```python
from build123d import *

# Parameters (mm, degrees)
BOSS_EXTRUDE1_DEPTH = 6.35
SKETCH2_R           = 2.4892
SKETCH2_R_2         = 4.7625
CUT_EXTRUDE1_DEPTH  = 7.35
FILLET1_R           = 6.35


with BuildPart() as part:
    # Sketch1 → Boss-Extrude1 (new body)
    with BuildSketch(Plane(origin=(0, 0, 0), x_dir=(1, 0, 0), z_dir=(0, 1, 0))):
        Polygon((0, 95.812682967), (85.38707615, 217.758065572), (127, 188.620382605), (127, 0), (0, 0), align=None)
    extrude(amount=BOSS_EXTRUDE1_DEPTH)

    # Sketch2 → Cut-Extrude1 (cut, through all)
    with BuildSketch(Plane(origin=(0, 6.35, 0), x_dir=(1, 0, 0), z_dir=(0, 1, 0))):
        with Locations((12.7, 12.7)):
            Circle(SKETCH2_R)
        with Locations((12.7, 38.1)):
            Circle(SKETCH2_R)
        with Locations((25.4, 38.1)):
            Circle(SKETCH2_R)
        with Locations((38.1, 38.1)):
            Circle(SKETCH2_R)
        with Locations((50.8, 38.1)):
            Circle(SKETCH2_R)
        with Locations((63.5, 38.1)):
            Circle(SKETCH2_R)
        with Locations((25.4, 12.7)):
            Circle(SKETCH2_R)
        with Locations((38.1, 12.7)):
            Circle(SKETCH2_R)
        with Locations((50.8, 12.7)):
            Circle(SKETCH2_R)
        with Locations((63.5, 12.7)):
            Circle(SKETCH2_R)
        with Locations((76.2, 12.7)):
            Circle(SKETCH2_R)
        with Locations((76.2, 38.1)):
            Circle(SKETCH2_R)
        with Locations((88.9, 12.7)):
            Circle(SKETCH2_R)
        with Locations((88.9, 38.1)):
            Circle(SKETCH2_R)
        with Locations((101.6, 12.7)):
            Circle(SKETCH2_R)
        with Locations((101.6, 38.1)):
            Circle(SKETCH2_R)
        with Locations((90.531859121, 202.963802812)):
            Circle(SKETCH2_R)
        with Locations((111.338321046, 188.394961329)):
            Circle(SKETCH2_R)
        with Locations((83.247438379, 192.56057185)):
            Circle(SKETCH2_R)
        with Locations((104.053900304, 177.991730366)):
            Circle(SKETCH2_R)
        with Locations((75.963017637, 182.157340887)):
            Circle(SKETCH2_R)
        with Locations((96.769479562, 167.588499404)):
            Circle(SKETCH2_R)
        with Locations((68.678596896, 171.754109925)):
            Circle(SKETCH2_R)
        with Locations((89.485058821, 157.185268441)):
            Circle(SKETCH2_R)
        with Locations((61.394176154, 161.350878962)):
            Circle(SKETCH2_R)
        with Locations((82.200638079, 146.782037479)):
            Circle(SKETCH2_R)
        with Locations((54.109755412, 150.947648)):
            Circle(SKETCH2_R)
        with Locations((74.916217337, 136.378806516)):
            Circle(SKETCH2_R)
        with Locations((46.825334671, 140.544417037)):
            Circle(SKETCH2_R)
        with Locations((67.631796596, 125.975575554)):
            Circle(SKETCH2_R)
        with Locations((39.540913929, 130.141186075)):
            Circle(SKETCH2_R)
        with Locations((60.347375854, 115.572344592)):
            Circle(SKETCH2_R)
        with Locations((17.687651704, 98.931493187)):
            Circle(SKETCH2_R_2)
        with Locations((28.090882667, 91.647072446)):
            Circle(SKETCH2_R_2)
        with Locations((38.494113629, 84.362651704)):
            Circle(SKETCH2_R_2)
        with Locations((114.3, 12.7)):
            Circle(SKETCH2_R)
        with Locations((114.3, 38.1)):
            Circle(SKETCH2_R)
    extrude(amount=-CUT_EXTRUDE1_DEPTH, mode=Mode.SUBTRACT)

    # Fillet1
    fillet1_edges = [part.edges().sort_by_distance(p)[0] for p in [
        (0, 3.175, -95.812682967),
        (85.38707615, 3.175, -217.758065572),
        (127, 3.175, -188.620382605),
        (127, 3.175, 0),
        (0, 3.175, 0),
    ]]
    fillet(fillet1_edges, radius=FILLET1_R)


solid = part.part
```
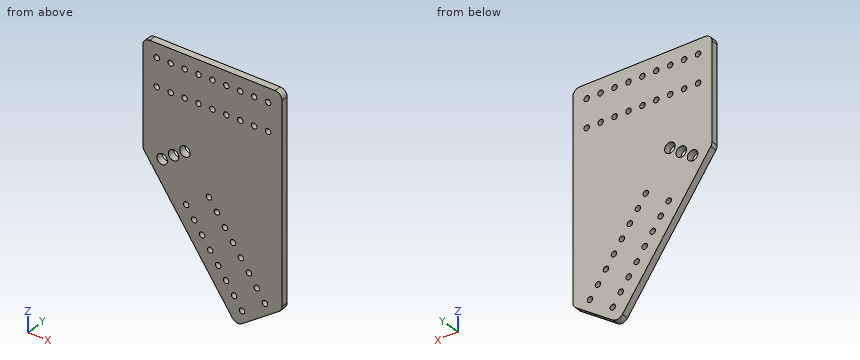
Can you work these out from the model? Positions are in its coordinate system, mm. Round coordinates to 2 decimals unless told otherwise and drop trailing zeros. Order: outer loops, then holes, each group sorted by start corner. A loop starts at its lowest first (then second) coordinate and runs counter-clockwise, first axis right, second up.
(1) If we section it at D-D (z = -108): Please give me the cut outline in (x, y).
Results are:
outline: (8.53, 0) - (127, 0) - (127, 6.35) - (8.53, 6.35) - close
(2) If we section it at B-B (z = -12.7): Count the separate pieces of the cut face and the enclosed holes in it, plus the area to 3 significant figures.
Results are:
separate pieces: 10
enclosed holes: 0
area: 522 mm2
(3) I'm going to push a flat-ended pin straight in: pin 1 (5.5 mm diameter, centred on x = 39.54, z = -130.14, fed in from +Y). Where does the tip first touch, or does it pass through?
Results are:
pin 1: stops at y = 6.35
(4) If I drill on L1, parallel to Z at x = 64.5, y = 5.5; L2, parallel to Z at x = 76.2, y = 2.75; L3, parallel to Z at x = 47, y = 0.75, over which ranges is the centre line in solid material (lowest first)?
Results are:
L1: z = -187.93 to -40.38, -35.82 to -14.98, -10.42 to 0
L2: z = -204.64 to -184.64, -179.68 to -138.51, -134.25 to -40.59, -35.61 to -15.19, -10.21 to 0
L3: z = -162.94 to -143.03, -138.06 to 0
(5) If we section it at A-A (x = 25.4): Please give me the cut outline in (y, z), plus the area to 3 significant figures.
Results are:
outline: (0, -132.09) - (6.35, -132.09) - (6.35, -95.58) - (0, -95.58) - close; (0, -87.72) - (6.35, -87.72) - (6.35, -40.59) - (0, -40.59) - close; (0, -35.61) - (6.35, -35.61) - (6.35, -15.19) - (0, -15.19) - close; (0, -10.21) - (6.35, -10.21) - (6.35, 0) - (0, 0) - close
area: 726 mm2
